Read the model definition and answer for the solid it produces. Units are mm, in the model's axes. Face numbers are marked on the shaded views. A direction names the side the tool comes from. Give positions to 0.01 mm unless a question says otherwise; leave off trailing zeros. Write each loop counter-clockwise with the first axis right and the second up, starting at its lowest first coordinate (ties: lowest second). Pieces come first, ordered by that corner, then holes. Notation, with made-up numbers: (85.25, 13) - (143.25, 13) arc R23 ccw to (143.25, 40) - close; hole circle Ø5 at (29.25, 8.5). An arc over 180 degrees is marked (long way). Answer as CSV lines item,"result".
```python
from build123d import *

# Parameters (mm, degrees)
ESQUISSE2_R                  = 8
BOSS_EXTRU_1_DEPTH           = 72
ESQUISSE3_R                  = 6
BOSS_EXTRU_2_DEPTH           = 4
ESQUISSE4_R                  = 9
BOSS_EXTRU_3_DEPTH           = 22
ESQUISSE5_R                  = 10
BOSS_EXTRU_4_DEPTH           = 3.5
ESQUISSE6_R                  = 9
BOSS_EXTRU_5_DEPTH           = 31.5
CHANFREIN1_SIZE              = 2
CHANFREIN2_SIZE              = 1
ENL_V_MAT_EXTRU_1_DEPTH      = 134.749766355
ENL_V_MAT_EXTRU_1_DEPTH_BACK = 134.749766355
ESQUISSE7_R                  = 5


with BuildPart() as part:
    # Esquisse2 → Boss.-Extru.1 (new body)
    with BuildSketch(Plane.XY):
        Circle(ESQUISSE2_R)
    extrude(amount=BOSS_EXTRU_1_DEPTH)

    # Esquisse3 → Boss.-Extru.2 (add)
    with BuildSketch(Plane.XY.offset(72)):
        Circle(ESQUISSE3_R)
    extrude(amount=BOSS_EXTRU_2_DEPTH)

    # Esquisse4 → Boss.-Extru.3 (add)
    with BuildSketch(Plane.XY.offset(76)):
        Circle(ESQUISSE4_R)
    extrude(amount=BOSS_EXTRU_3_DEPTH)

    # Esquisse5 → Boss.-Extru.4 (add)
    with BuildSketch(Plane.XY.offset(98)):
        Circle(ESQUISSE5_R)
    extrude(amount=BOSS_EXTRU_4_DEPTH)

    # Esquisse6 → Boss.-Extru.5 (add)
    with BuildSketch(Plane.XY.offset(101.5)):
        Circle(ESQUISSE6_R)
    extrude(amount=BOSS_EXTRU_5_DEPTH)

    # Chanfrein1
    chanfrein1_edges = [part.edges().sort_by_distance(p)[0] for p in [
        (-9, 0, 133),
    ]]
    chamfer(chanfrein1_edges, length=CHANFREIN1_SIZE)

    # Chanfrein2
    chanfrein2_edges = [part.edges().sort_by_distance(p)[0] for p in [
        (-8, 0, 0),
    ]]
    chamfer(chanfrein2_edges, length=CHANFREIN2_SIZE)

    # Esquisse7 → Enlèv. mat.-Extru.1 (cut, two sides: drawn at the far end of the back side and taken through both)
    with BuildSketch(Plane(origin=(0, 0, 0), x_dir=(1, 0, 0), z_dir=(0, 1, 0)).offset(-ENL_V_MAT_EXTRU_1_DEPTH_BACK)):
        with Locations(Location((0, -121, 0), (0, 0, 270))):
            Circle(ESQUISSE7_R)
    extrude(amount=ENL_V_MAT_EXTRU_1_DEPTH + ENL_V_MAT_EXTRU_1_DEPTH_BACK, mode=Mode.SUBTRACT)


solid = part.part
```
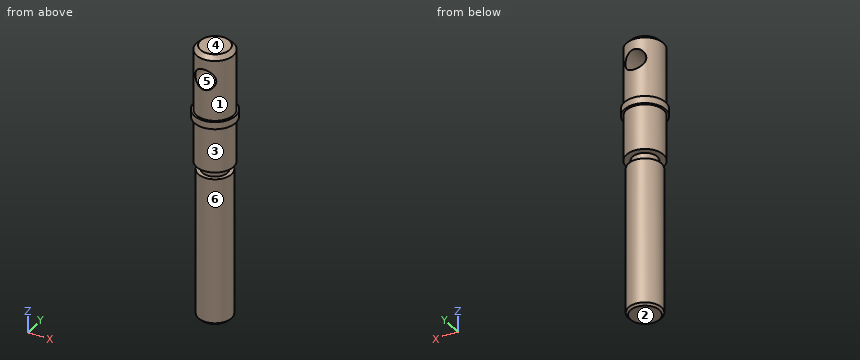
(1) A cutting plane is placed at B-B (y = 0). Write down the section's boundary in (x, z).
Worked out:
outline,"(-10, 98) - (-9, 98) - (-9, 76) - (-6, 76) - (-6, 72) - (-8, 72) - (-8, 1) - (-7, 0) - (7, 0) - (8, 1) - (8, 72) - (6, 72) - (6, 76) - (9, 76) - (9, 98) - (10, 98) - (10, 101.5) - (9, 101.5) - (9, 131) - (7, 133) - (-7, 133) - (-9, 131) - (-9, 101.5) - (-10, 101.5) - close; hole circle Ø10 at (0, 121)"
(2) Each of these flat-tipped pins is pushed along its axis until it touches: P1, Ø5, axis at y = -4, z = 110, coming from the -X side; P2, Ø5, axis at y = -7.5, z = 31.5, coming from the -X side (3 decimals); P3, Ø11.5, axis at x = 0, z = 121, coming from the +Y side. Where does it stop, or does it pass through?
Worked out:
P1,"stops at x = -8.87"
P2,"stops at x = -6.245"
P3,"stops at y = 9"
(3) A cutting plane is placed at C-C (z = 121). Write down the section's boundary in (x, y).
Worked out:
outline,"(-5, -7.48) - (-5, 7.48) arc R9 ccw to start; (5, -7.48) arc R9 ccw to (5, 7.48) - close"
(4) A cutting plane is placed at D-D (z = 103.5). Write down the section's boundary in (x, y), and give its area (3 significant figures).
Worked out:
outline,"circle Ø18 at (0, 0)"
area,"254 mm^2"
(5) Find the intervals of material crossed by L1, parallel to Z at x = -0.25, y = -7; L2, parallel to Z at x = 0, y = -1.25; L3, parallel to Z at x = 1.75, y = 6.25, in increasing order.
Worked out:
L1,"z = 0 to 72, 76 to 116.01, 125.99 to 133"
L2,"z = 0 to 116, 126 to 133"
L3,"z = 0 to 72, 76 to 116.32, 125.68 to 133"
(6) A cutting plane is placed at A-A (x = 0). Write down the section's boundary in (y, z), and give its area (3 significant figures).
Worked out:
outline,"(-10, 98) - (-9, 98) - (-9, 76) - (-6, 76) - (-6, 72) - (-8, 72) - (-8, 1) - (-7, 0) - (7, 0) - (8, 1) - (8, 72) - (6, 72) - (6, 76) - (9, 76) - (9, 98) - (10, 98) - (10, 101.5) - (9, 101.5) - (9, 116) - (-9, 116) - (-9, 101.5) - (-10, 101.5) - close; (-9, 126) - (9, 126) - (9, 131) - (7, 133) - (-7, 133) - (-9, 131) - close"
area,"2,050 mm^2"
(7) The mould has two halves that part along Z. Classify the marked faces 4, 5 and 6: +Z half, -Z half, draft (parallel to the pull), parting line (faces both ways), or undercut.
Worked out:
face 4,"+Z half"
face 5,"undercut"
face 6,"draft"
(8) For the marked faces 1, 2 and 3, determine the directions among +Z, -Z, +X, -X, +Y, -Y from which every point of the face is accessible in a straight line to the end or side of a thin tool.
Worked out:
face 1,"+Z"
face 2,"-Z, +X, -X, +Y, -Y"
face 3,"-Z"
